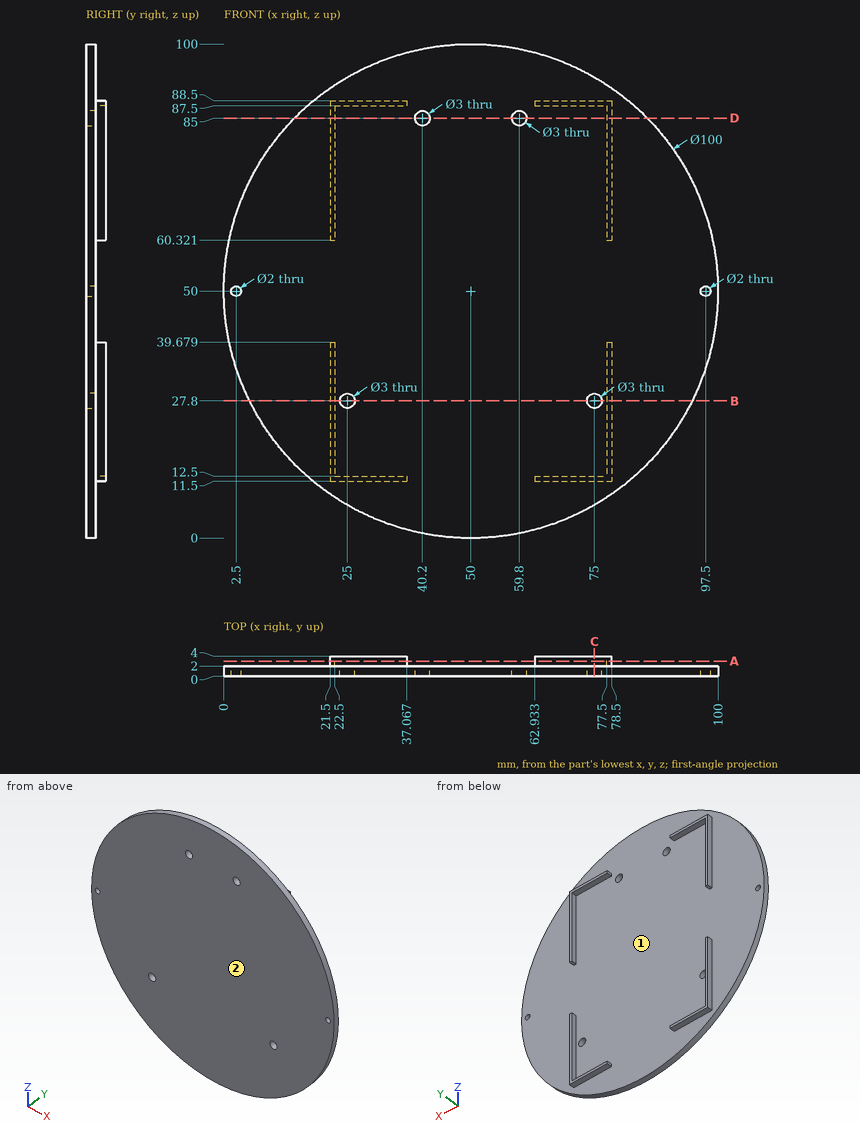
Answer from the drawing. Dimensions are ordinates in mm from the lowest x, y and z of the part. Round coordinates to 2 decimals unless told otherwise and drop trailing zeros. Write each loop counter-clockwise with the first axis right and the second up, starting at its lowest first coordinate (ties: lowest second). Pieces come first, ordered by that corner, then holes.
1. The part is cut by section C-C, the plane x = 75. Determine the outline of the cut face in (y, z), then the cut area to 3 significant figures.
2. Straight lines are drawn through the part: L1, parallel to X at y = 3, z = 18; L2, parallel to Z at x = 32.5, y = 3.65; L3, parallel to X at y = 0.65, z = 27.8. For each, find the intervals that lie inside material, in ascending order.
3. Determine the mould class of the marked faces 1 and 2 for opening direction Z: pulls with the +Z half, pulls with the -Z half, needs draft (parallel to the pull), parting line crosses it, or undercut.
4. The part is cut by section B-B, the plane z = 27.8. Determine the outline of the cut face in (x, y).
5. The part is cut by section D-D, the plane z = 85. Determine the outline of the cut face in (x, y).
6. Given pin 1 Ø0.6 at (y, z) = (2.5, 26) entering from +X; pin 2 Ø1.6 at (x, y) = (31.5, 2.5) entering from -Z; pin 3 Ø1 at (x, y) = (26, 3) entering from +Z, each flat-ended and moving along its own axis, determine where each tip first touches the part or whether it passes through.
7. The part is cut by section A-A, the plane y = 3. Determine the outline of the cut face in (x, z).
Values:
1. outline: (0, 6.7) - (2, 6.7) - (2, 11.5) - (4, 11.5) - (4, 12.5) - (2, 12.5) - (2, 26.3) - (0, 26.3) - close; (0, 29.3) - (2, 29.3) - (2, 87.5) - (4, 87.5) - (4, 88.5) - (2, 88.5) - (2, 93.3) - (0, 93.3) - close
1. area: 171 mm2
2. L1: x = 21.5 to 22.5, 77.5 to 78.5
2. L2: z = 11.5 to 12.5, 87.5 to 88.5
2. L3: x = 5.2 to 23.5, 26.5 to 73.5, 76.5 to 94.8
3. face 1: undercut
3. face 2: needs draft
4. outline: (5.2, 0) - (23.5, 0) - (23.5, 2) - (22.5, 2) - (22.5, 4) - (21.5, 4) - (21.5, 2) - (5.2, 2) - close; (26.5, 0) - (73.5, 0) - (73.5, 2) - (26.5, 2) - close; (76.5, 0) - (94.8, 0) - (94.8, 2) - (78.5, 2) - (78.5, 4) - (77.5, 4) - (77.5, 2) - (76.5, 2) - close
5. outline: (14.29, 0) - (38.7, 0) - (38.7, 2) - (22.5, 2) - (22.5, 4) - (21.5, 4) - (21.5, 2) - (14.29, 2) - close; (41.7, 0) - (58.3, 0) - (58.3, 2) - (41.7, 2) - close; (61.3, 0) - (85.71, 0) - (85.71, 2) - (78.5, 2) - (78.5, 4) - (77.5, 4) - (77.5, 2) - (61.3, 2) - close
6. pin 1: stops at x = 78.5
6. pin 2: stops at z = 3.3
6. pin 3: stops at z = 88.5
7. outline: (21.5, 11.5) - (37.07, 11.5) - (37.07, 12.5) - (22.5, 12.5) - (22.5, 39.68) - (21.5, 39.68) - close; (21.5, 60.32) - (22.5, 60.32) - (22.5, 87.5) - (37.07, 87.5) - (37.07, 88.5) - (21.5, 88.5) - close; (62.93, 11.5) - (78.5, 11.5) - (78.5, 39.68) - (77.5, 39.68) - (77.5, 12.5) - (62.93, 12.5) - close; (62.93, 87.5) - (77.5, 87.5) - (77.5, 60.32) - (78.5, 60.32) - (78.5, 88.5) - (62.93, 88.5) - close
